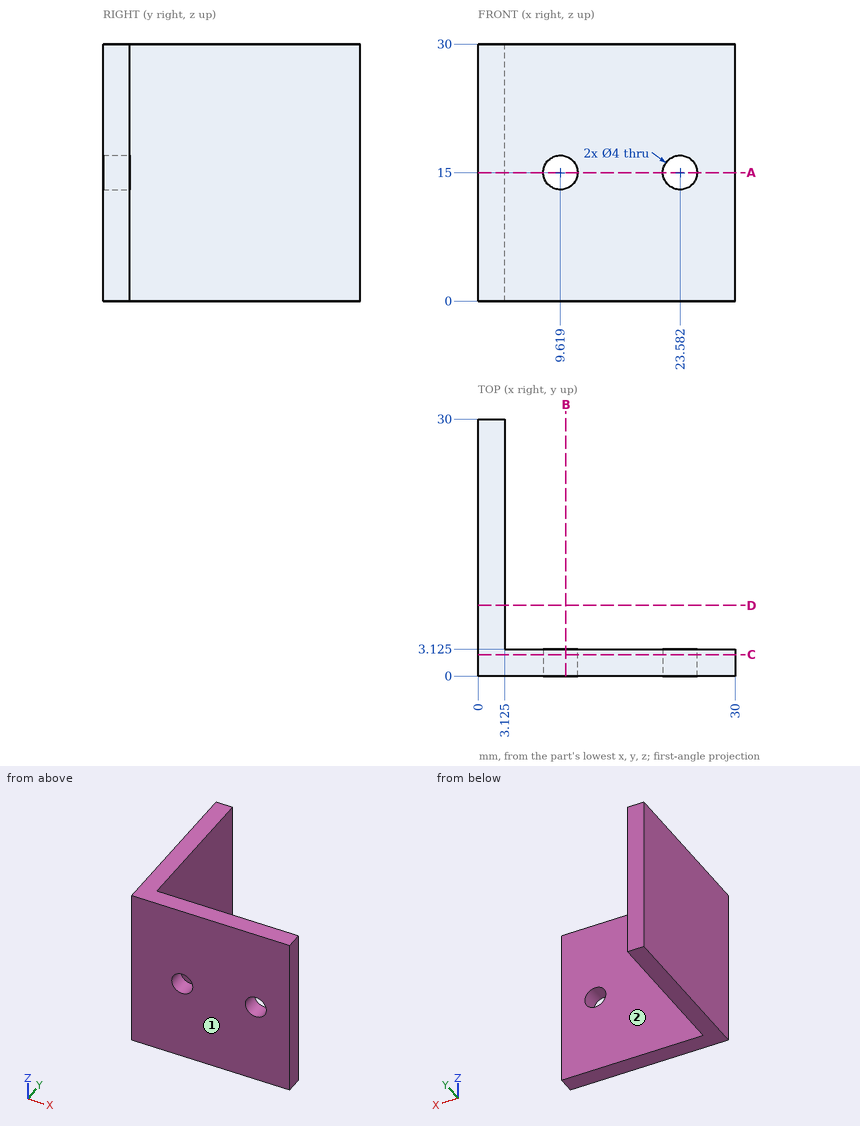
Geometry check sheet. Reference: drawing and pictorial views, mm from the part's lowest x, y, z. A direction names the side the tool comes from. Round coordinates to 2 decimals unless told otherwise and drop trailing zeros. Loops run counter-clockwise (first coordinate to the right, second up) from the corner with the lowest first, then second, coordinate; pieces in that order, holes last. Notation, with made-up numbers: (78.25, 27.25) - (117.25, 27.25) arc R30 cw to (117.25, 55.25) - close; hole circle Ø2 at (-16.5, -5). An arc over 180 degrees is marked (long way). One line per question, with ' | ' between items. Start each with the question number.
1. Cross-section at D-D on y = 8.25. Record the cut outline in (x, z) (1 decimal).
2. Scan line: line 1 (Y direction, x = 8.5, z = 20) (1 decimal). Record every from-to range of solid material in increasing order. Write a range as [from, to].
3. Depth check by flat-ended pin: pin 1 (6.5 mm diameter, centred on x = 23.58, z = 15, fed in from +Y) (3 decimals). Enter the tip coordinate at first touch or a pass-through.
4. Tool access check on the marked faces 1 and 2. Record the directions out of +Z, -Z, +X, -X, +Y, -Y that give a thin tool (end or side, any length) a straight path to the whole face; none if there is none.
5. Cross-section at C-C on y = 2.5. Record the cut outline in (x, z), then the cut area to 3 significant figures.
6. Cross-section at B-B on x = 10.25. Record the cut outline in (y, z) (1 decimal).
7. Cross-section at A-A on z = 15. Record the cut outline in (x, y) (1 decimal).
Taken from the geometry:
1) outline: (0, 0) - (3.1, 0) - (3.1, 30) - (0, 30) - close
2) line 1: [0, 3.1]
3) pin 1: y = 3.125
4) face 1: +Z, -Z, +X, -X, -Y | face 2: +Z, -Z, +X, +Y
5) outline: (0, 0) - (30, 0) - (30, 30) - (0, 30) - close; hole circle Ø4 at (9.62, 15); hole circle Ø4 at (23.58, 15) | area: 875 mm²
6) outline: (0, 0) - (3.1, 0) - (3.1, 13.1) - (0, 13.1) - close; (0, 16.9) - (3.1, 16.9) - (3.1, 30) - (0, 30) - close
7) outline: (0, 0) - (7.6, 0) - (7.6, 3.1) - (3.1, 3.1) - (3.1, 30) - (0, 30) - close; (11.6, 0) - (21.6, 0) - (21.6, 3.1) - (11.6, 3.1) - close; (25.6, 0) - (30, 0) - (30, 3.1) - (25.6, 3.1) - close
